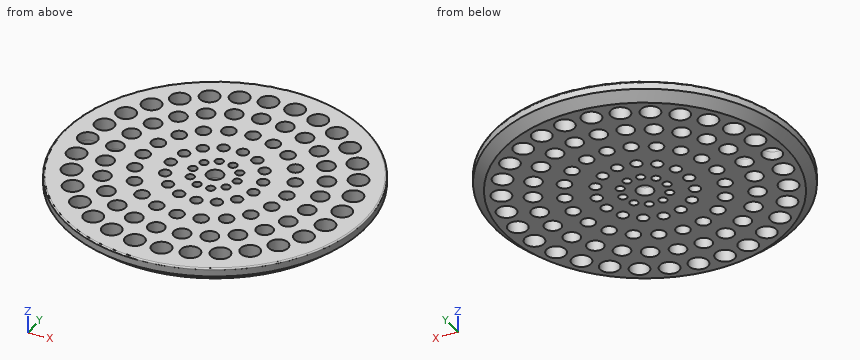
from build123d import *

# Parameters (mm, degrees)
SKETCH020_R           = 3.5
POCKET008_DEPTH       = 100
POCKET008_DEPTH_BACK  = 100
SKETCH021_R           = 3
POCKET009_DEPTH       = 100
POCKET009_DEPTH_BACK  = 100
SKETCH022_R           = 2.5
POCKET010_DEPTH       = 100
POCKET010_DEPTH_BACK  = 100
SKETCH023_R           = 2
POCKET011_DEPTH       = 100
POCKET011_DEPTH_BACK  = 100
SKETCH024_R           = 1.5
POCKET012_DEPTH       = 100
POCKET012_DEPTH_BACK  = 100
SKETCH025_R           = 3
POCKET013_DEPTH       = 100
POCKET013_DEPTH_BACK  = 100
POLARPATTERN005_COUNT = 30
POLARPATTERN006_COUNT = 25
POLARPATTERN007_COUNT = 20
POLARPATTERN008_COUNT = 15
POLARPATTERN009_COUNT = 10
FILLET_R              = 0.5


with BuildPart() as part:
    # Sketch003 → Revolution001 (revolve)
    with BuildSketch(Plane.XZ):
        Polygon((0, 3), (-55, 3), (-55, 0), (-51.5, -3), (0, -3), align=None)
    revolve(axis=Axis((0, 0, 0), (0, 0, 1)))

    # Sketch020 → Pocket008 (cut, two sides)
    with BuildSketch(Plane.XY) as pocket008_sk:
        with Locations((-46, 0)):
            Circle(SKETCH020_R)
    pocket008 = extrude(amount=-POCKET008_DEPTH, mode=Mode.SUBTRACT) + extrude(pocket008_sk.sketch, amount=POCKET008_DEPTH_BACK, mode=Mode.SUBTRACT)

    # Sketch021 → Pocket009 (cut, two sides)
    with BuildSketch(Plane.XY) as pocket009_sk:
        with Locations((-36, 0)):
            Circle(SKETCH021_R)
    pocket009 = extrude(amount=-POCKET009_DEPTH, mode=Mode.SUBTRACT) + extrude(pocket009_sk.sketch, amount=POCKET009_DEPTH_BACK, mode=Mode.SUBTRACT)

    # Sketch022 → Pocket010 (cut, two sides)
    with BuildSketch(Plane.XY) as pocket010_sk:
        with Locations((-26, 0)):
            Circle(SKETCH022_R)
    pocket010 = extrude(amount=-POCKET010_DEPTH, mode=Mode.SUBTRACT) + extrude(pocket010_sk.sketch, amount=POCKET010_DEPTH_BACK, mode=Mode.SUBTRACT)

    # Sketch023 → Pocket011 (cut, two sides)
    with BuildSketch(Plane.XY) as pocket011_sk:
        with Locations((-16, 0)):
            Circle(SKETCH023_R)
    pocket011 = extrude(amount=-POCKET011_DEPTH, mode=Mode.SUBTRACT) + extrude(pocket011_sk.sketch, amount=POCKET011_DEPTH_BACK, mode=Mode.SUBTRACT)

    # Sketch024 → Pocket012 (cut, two sides)
    with BuildSketch(Plane.XY) as pocket012_sk:
        with Locations((-8, 0)):
            Circle(SKETCH024_R)
    pocket012 = extrude(amount=-POCKET012_DEPTH, mode=Mode.SUBTRACT) + extrude(pocket012_sk.sketch, amount=POCKET012_DEPTH_BACK, mode=Mode.SUBTRACT)

    # Sketch025 → Pocket013 (cut, two sides)
    with BuildSketch(Plane.XY) as pocket013_sk:
        Circle(SKETCH025_R)
    extrude(amount=-POCKET013_DEPTH, mode=Mode.SUBTRACT)
    extrude(pocket013_sk.sketch, amount=POCKET013_DEPTH_BACK, mode=Mode.SUBTRACT)

    # PolarPattern005: Pocket008 ×30 about axis
    polarpattern005_axis = Axis((0, 0, 0), (0, 0, 1))
    for i in range(1, POLARPATTERN005_COUNT):
        add(pocket008.rotate(polarpattern005_axis, i * 360 / POLARPATTERN005_COUNT), mode=Mode.SUBTRACT)

    # PolarPattern006: Pocket009 ×25 about axis
    polarpattern006_axis = Axis((0, 0, 0), (0, 0, 1))
    for i in range(1, POLARPATTERN006_COUNT):
        add(pocket009.rotate(polarpattern006_axis, i * 360 / POLARPATTERN006_COUNT), mode=Mode.SUBTRACT)

    # PolarPattern007: Pocket010 ×20 about axis
    polarpattern007_axis = Axis((0, 0, 0), (0, 0, 1))
    for i in range(1, POLARPATTERN007_COUNT):
        add(pocket010.rotate(polarpattern007_axis, i * 360 / POLARPATTERN007_COUNT), mode=Mode.SUBTRACT)

    # PolarPattern008: Pocket011 ×15 about axis
    polarpattern008_axis = Axis((0, 0, 0), (0, 0, 1))
    for i in range(1, POLARPATTERN008_COUNT):
        add(pocket011.rotate(polarpattern008_axis, i * 360 / POLARPATTERN008_COUNT), mode=Mode.SUBTRACT)

    # PolarPattern009: Pocket012 ×10 about axis
    polarpattern009_axis = Axis((0, 0, 0), (0, 0, 1))
    for i in range(1, POLARPATTERN009_COUNT):
        add(pocket012.rotate(polarpattern009_axis, i * 360 / POLARPATTERN009_COUNT), mode=Mode.SUBTRACT)

    # Fillet
    fillet_edges = [part.edges().sort_by_distance(p)[0] for p in [
        (55, 0, 3),
    ]]
    fillet(fillet_edges, radius=FILLET_R)


solid = part.part
Design review of the part built by this model. Coordinates are the model's own, in mm. Round coordinates to 2 decimals unless told otherwise and drop trailing zeros. Answer as a JSON object with one key per item and string values.
Item 1: Wall thickness on L1, parallel to Y at x = -27, z = -2.25; L2, parallel to Y at x = 45, z = 0.5; L3, parallel to X at y = 5, z = -0.25: over which ranges is each line inside the solid? List them lowest first. Write a range as from..to.
Answer sheet:
{"L1": "y = -44.88..-27.55, -21.74..-9.08, -6.99..-2.29, 2.29..6.99, 9.08..21.74, 27.55..44.88", "L2": "y = -31.62..-20.55, -16.87..-13.06, -6.06..-3.35, 3.35..6.06, 13.06..16.87, 20.55..31.62", "L3": "x = -54.48..-15.93, -13.3..-7.94, -5..5, 7.94..14.56, 16.75..32.76, 38.68..54.48"}
Item 2: Clearance check with flat-ended pins moving along their axes: P1, Ø2, axis at y = -7, z = -0.5, coming from the -X side; P2, Ø1, axis at y = -5, z = 2, coming from the -X side; P3, Ø1, axis at y = 32.5, z = 0, coming from the +X side. State where each tip first meets the part, or that it passes through.
Answer sheet:
{"P1": "stops at x = -54.66", "P2": "stops at x = -54.82", "P3": "stops at x = 44.73"}
Item 3: We need section A-A on x = -36. State how many separate pieces and enclosed holes the cut face has, and give its area (3 significant figures).
Answer sheet:
{"separate pieces": "6", "enclosed holes": "0", "area": "303 mm^2"}
